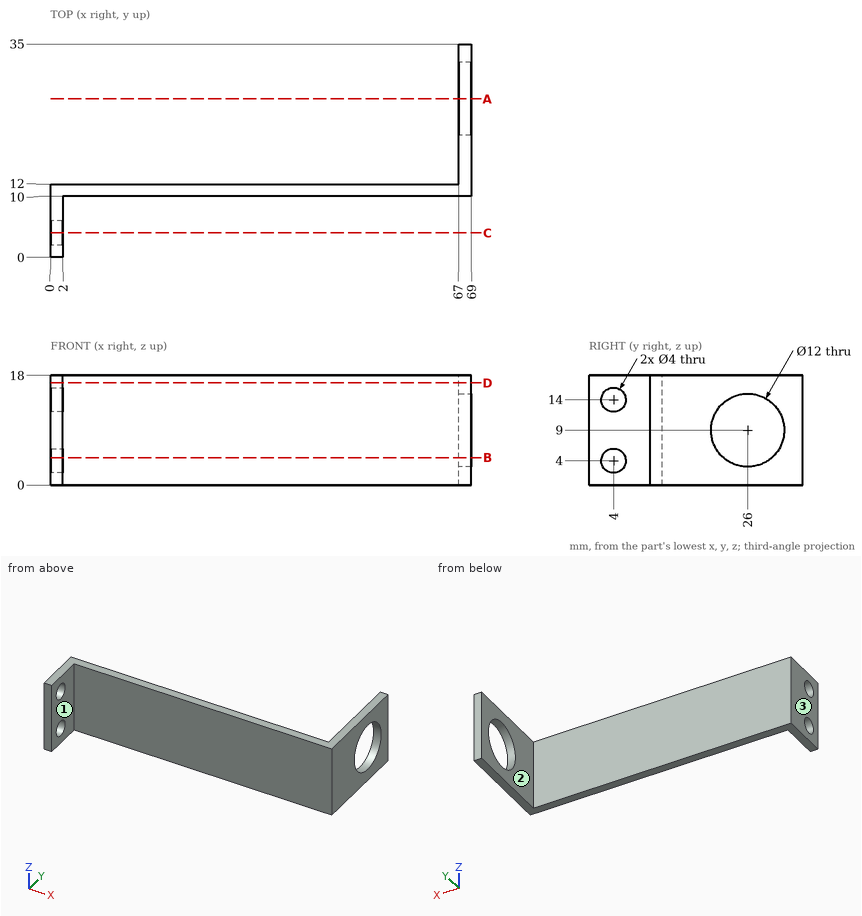
The drawing under review shows one solid part. Ordinate dimensions are in mm from its lowest x, y, z. A direction names the side the tool comes from. Round coordinates to 2 decimals unless told otherwise and drop trailing zeros. Loops run counter-clockwise (first coordinate to the right, second up) from the corner with the lowest first, then second, coordinate; pieces in that order, holes last. Notation, with made-up numbers: (-35, 22.25) - (4, 22.25) arc R19 cw to (4, 40.25) - close; hole circle Ø1 at (83.5, -36.75). An arc over 180 degrees is marked (long way). One line per question, with ' | ' between items.
Q1. For pin 1 (1 mm diameter, centred on x = 51, z = 7, fed in from +Y); pin 2 (8 mm diameter, centred on y = 5, z = 8, fed in from +X), all flat-tipped, find the tip position at first contact; note any pin that passes through.
Taken from the geometry:
pin 1: stops at y = 12 | pin 2: stops at x = 2
Q2. Tool access review of the marked faces 1, 2 and 3: name each direction out of +Z, -Z, +X, -X, +Y, -Y from which nothing blocks a thin tool from reaching the whole face with its end or side.
Taken from the geometry:
face 1: +Z, -Z, +X, -Y | face 2: +Z, -Z, -X, +Y | face 3: +Z, -Z, -X, +Y, -Y
Q3. Take a section at D-D (z = 16.75). Give the boundary of the cut face in (x, y).
Taken from the geometry:
outline: (0, 0) - (2, 0) - (2, 10) - (69, 10) - (69, 35) - (67, 35) - (67, 12) - (0, 12) - close
Q4. Take a section at A-A (y = 26). Give the boundary of the cut face in (x, z).
Taken from the geometry:
outline: (67, 0) - (69, 0) - (69, 3) - (67, 3) - close; (67, 15) - (69, 15) - (69, 18) - (67, 18) - close
Q5. Take a section at B-B (z = 4.5). Give the boundary of the cut face in (x, y).
Taken from the geometry:
outline: (0, 0) - (2, 0) - (2, 2.06) - (0, 2.06) - close; (0, 5.94) - (2, 5.94) - (2, 10) - (69, 10) - (69, 22.03) - (67, 22.03) - (67, 12) - (0, 12) - close; (67, 29.97) - (69, 29.97) - (69, 35) - (67, 35) - close
Q6. Take a section at C-C (y = 4). Give the boundary of the cut face in (x, z).
Taken from the geometry:
outline: (0, 0) - (2, 0) - (2, 2) - (0, 2) - close; (0, 6) - (2, 6) - (2, 12) - (0, 12) - close; (0, 16) - (2, 16) - (2, 18) - (0, 18) - close
Q7. For line 1 along Y through (x, z) = (1.45, 4); line 2 along Y through (x, z) = (67.85, 9); line 3 along Y through (x, z) = (19, 6), list the stretches that pass through material, from the lowest coordinate up. Write a range as [from, to].
Taken from the geometry:
line 1: y = [0, 2], [6, 12] | line 2: y = [10, 20], [32, 35] | line 3: y = [10, 12]
